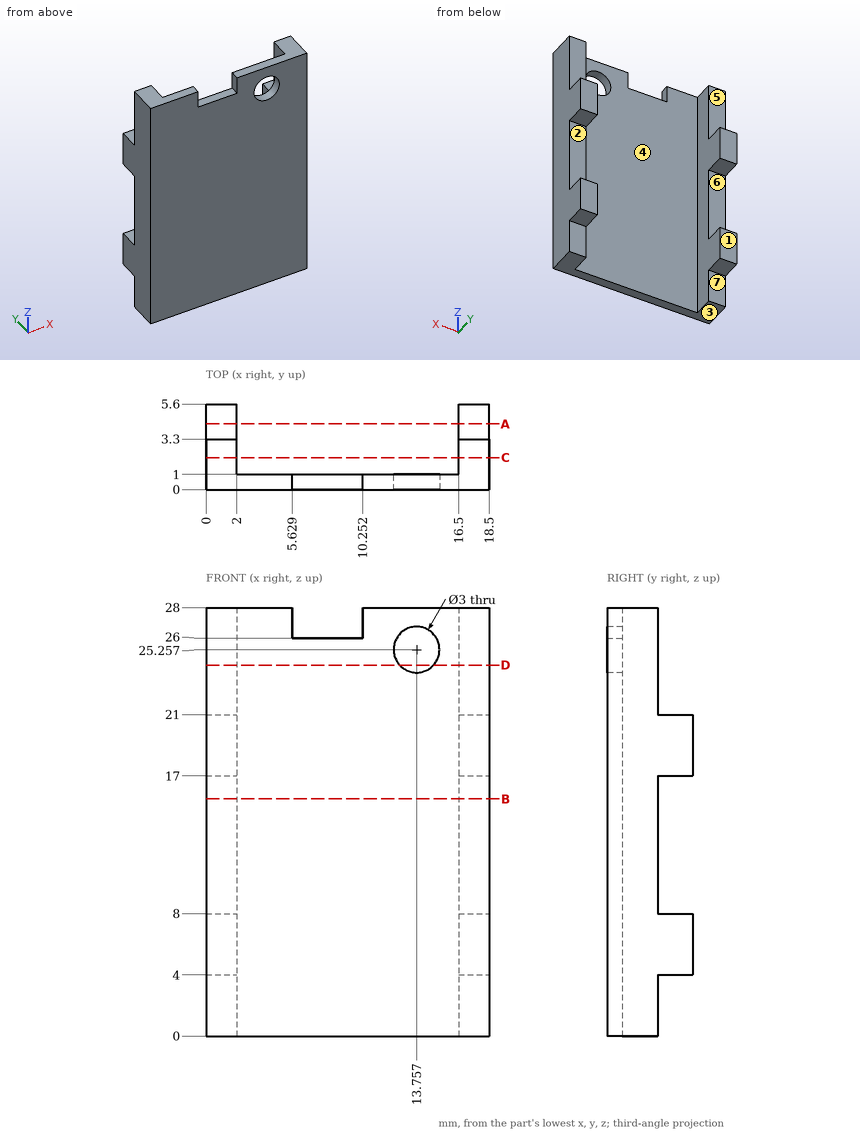
Here's the drawing with two shaded views (mm, measured from the low corner). I have some questions. A direction names the side the tool comes from. Round coordinates to 2 decimals unless told otherwise and drop trailing zeros. Loops run counter-clockwise (first coordinate to the right, second up) from the corner with the lowest first, then second, coordinate; pieces in that order, holes last. Notation, with made-up numbers: (19.25, 18.5) -> (61.25, 18.5) arc R16 cw to (61.25, 22.5) -> close; hole circle Ø3 at (-26.75, 34). An arc over 180 degrees is marked (long way). Answer as CSV lines item,"result". Start each with the question number.
1. Imagine slicing it at A-A on y = 4.3. Write out the boundary of the cut face in (x, z), plus the area to 3 significant figures.
2. Imagine slicing it at B-B on z = 15.5. Write out the boundary of the cut face in (x, y), plus the area to 3 significant figures.
3. I'm going to push flat-ended pins straight in: P1, Ø1.6, axis at x = 17.5, z = 11.5, coming from the +Y side; P2, Ø1.8, axis at x = 13.76, z = 25.26, coming from the -Y side; P3, Ø0.5, axis at x = 7, y = 0.5, coming from the +Z side; P4, Ø0.6, axis at x = 18, y = 4, coming from the -Z side. Where does each tip first touch, or does it pass through?
4. Imagine slicing it at C-C on y = 2.1. Write out the boundary of the cut face in (x, z), plus the area to 3 significant figures.
5. Imagine slicing it at D-D on z = 24.25. Write out the boundary of the cut face in (x, y) (1 decimal).
6. If we mould it in two halves opening along Z, with no side actions, what happens to the marked faces 1, 2 and 3? For each: pulls with the +Z half, pulls with the -Z half, needs draft (parallel to the pull), parting line crosses it, or undercut.
7. For the marked faces 4, 5, 6 and 7, which set-ups out of +Z, -Z, +X, -X, +Y, -Y let a thin tool reach every point of the face, with its end or its side?
8. I need wall thicknesses on probe 1 along X at (y, z) = (1.65, 24.25); probe 2 along Y at (x, z) = (11.5, 18.25); probe 3 along Z at (x, y) = (7.75, 0.95). Which ranges of each line are inside material? Lowest first, please. Write a range as from..to.
Solution:
1,outline,"(0, 4) -> (2, 4) -> (2, 8) -> (0, 8) -> close; (0, 17) -> (2, 17) -> (2, 21) -> (0, 21) -> close; (16.5, 4) -> (18.5, 4) -> (18.5, 8) -> (16.5, 8) -> close; (16.5, 17) -> (18.5, 17) -> (18.5, 21) -> (16.5, 21) -> close"
1,area,"32.0 mm²"
2,outline,"(0, 0) -> (18.5, 0) -> (18.5, 3.3) -> (16.5, 3.3) -> (16.5, 1) -> (2, 1) -> (2, 3.3) -> (0, 3.3) -> close"
2,area,"27.7 mm²"
3,P1,"y = 3.3"
3,P2,"through"
3,P3,"z = 26"
3,P4,"z = 4"
4,outline,"(0, 0) -> (2, 0) -> (2, 28) -> (0, 28) -> close; (16.5, 0) -> (18.5, 0) -> (18.5, 28) -> (16.5, 28) -> close"
4,area,"112 mm²"
5,outline,"(0, 0) -> (12.6, 0) -> (12.6, 1) -> (2, 1) -> (2, 3.3) -> (0, 3.3) -> close; (14.9, 0) -> (18.5, 0) -> (18.5, 3.3) -> (16.5, 3.3) -> (16.5, 1) -> (14.9, 1) -> close"
6,face 1,"needs draft"
6,face 2,"undercut"
6,face 3,"pulls with the -Z half"
7,face 4,"+Z, -Z, +Y"
7,face 5,"+Z, +X, -X, +Y"
7,face 6,"+X, -X, +Y"
7,face 7,"-Z, +X, -X, +Y"
8,probe 1,"0..2, 16.5..18.5"
8,probe 2,"0..1"
8,probe 3,"0..26"
